```python
from build123d import *

# Parameters (mm, degrees)
SKETCH1_W           = 17.5768
SKETCH1_H           = 11.176
BOSS_EXTRUDE1_DEPTH = 24.13
CUT_EXTRUDE1_DEPTH  = 22.55
SKETCH3_W           = 2.3304
SKETCH3_H           = 3.81
SKETCH3_W_2         = 2.2288
SKETCH3_H_2         = 3.7084
CUT_EXTRUDE2_DEPTH  = 0.254


with BuildPart() as part:
    # Sketch1 → Boss-Extrude1 (new body)
    with BuildSketch(Plane.XY):
        with Locations((8.7884, 5.588)):
            Rectangle(SKETCH1_W, SKETCH1_H)
    extrude(amount=-BOSS_EXTRUDE1_DEPTH)

    # Sketch2 → Cut-Extrude1 (cut)
    with BuildSketch(Plane.XY):
        Polygon((2.8384, 1.628), (14.7384, 1.628), (14.7384, 8.228), (11.9634, 8.228), (11.9634, 9.098), (10.8184, 9.098), (10.8184, 9.548), (6.7584, 9.548), (6.7584, 9.098), (5.6134, 9.098), (5.6134, 8.228), (2.8384, 8.228), align=None)
    extrude(amount=-CUT_EXTRUDE1_DEPTH, mode=Mode.SUBTRACT)

    # Sketch3 → Cut-Extrude2 (cut)
    with BuildSketch(Plane.XY):
        with Locations((1.4192, 8.636)):
            Rectangle(SKETCH3_W, SKETCH3_H)
        with Locations((1.4192, 8.636)):
            Rectangle(SKETCH3_W_2, SKETCH3_H_2, mode=Mode.SUBTRACT)
        with Locations((16.1576, 8.636)):
            Rectangle(SKETCH3_W, SKETCH3_H)
        with Locations((16.1576, 8.636)):
            Rectangle(SKETCH3_W_2, SKETCH3_H_2, mode=Mode.SUBTRACT)
    extrude(amount=-CUT_EXTRUDE2_DEPTH, mode=Mode.SUBTRACT)


solid = part.part
```
Source: CAD feature listing. Evaluate the final solid. Frame: model axes, mm. A direction names the side the tool comes from. Coordinates: 2 decimals unless noted, no trailing zeros. Order: outer loops, then holes, each group sorted by start corner. A loop starts at its lowest first (then second) coordinate and runs counter-clockwise, first axis right, second up. Notation, with made-up numbers: (12, 0) - (52, 0) arc R15 cw to (52, 15) - close; hole circle Ø1 at (4, -12). An arc over 180 degrees is marked (long way). One line per item, written item: value.
1) Ray query, line 1 (Y direction, x = 8.75, z = -8); line 2 (Y direction, x = 12.75, z = -17.5); line 3 (X direction, y = 5.5, z = -18.5). Return the intervals inside material, ascending. Write a range as [from, to].
Computed values:
line 1: y = [0, 1.63], [9.55, 11.18]
line 2: y = [0, 1.63], [8.23, 11.18]
line 3: x = [0, 2.84], [14.74, 17.58]
2) Cut plane A-A on z = -20.25. Output: boundary loops of the cut face in (x, y).
Computed values:
outline: (0, 0) - (17.58, 0) - (17.58, 11.18) - (0, 11.18) - close; hole (2.84, 1.63) - (14.74, 1.63) - (14.74, 8.23) - (11.96, 8.23) - (11.96, 9.1) - (10.82, 9.1) - (10.82, 9.55) - (6.76, 9.55) - (6.76, 9.1) - (5.61, 9.1) - (5.61, 8.23) - (2.84, 8.23) - close
3) Cut plane B-B on y = 8.5. Output: boundary loops of the cut face in (x, z).
Computed values:
outline: (0, -24.13) - (17.58, -24.13) - (17.58, 0) - (17.32, 0) - (17.32, -0.25) - (17.27, -0.25) - (17.27, 0) - (15.04, 0) - (15.04, -0.25) - (14.99, -0.25) - (14.99, 0) - (11.96, 0) - (11.96, -22.55) - (5.61, -22.55) - (5.61, 0) - (2.58, 0) - (2.58, -0.25) - (2.53, -0.25) - (2.53, 0) - (0.3, 0) - (0.3, -0.25) - (0.25, -0.25) - (0.25, 0) - (0, 0) - close
4) Cut plane D-D on y = 2.5. Output: boundary loops of the cut face in (x, z), plus the area to 3 significant figures.
Computed values:
outline: (0, -24.13) - (17.58, -24.13) - (17.58, 0) - (14.74, 0) - (14.74, -22.55) - (2.84, -22.55) - (2.84, 0) - (0, 0) - close
area: 156 mm^2
5) Reachability of faces 4 (the face through (16, 9, 0)), 5 (the face through (2.838, 5, -11)) from +Z, -Z, +X, -X, +Y, -Y: full face, straight path, thin tool, end or side. Return the list, or none.
Computed values:
face 4: +Z, +X, -X, +Y, -Y
face 5: +Z
6) Cut plane C-C on x = 11.5. Output: boundary loops of the cut face in (y, z).
Computed values:
outline: (0, -24.13) - (11.18, -24.13) - (11.18, 0) - (9.1, 0) - (9.1, -22.55) - (1.63, -22.55) - (1.63, 0) - (0, 0) - close
7) Mould query, pull axis Y, two halves, no side actions, for faces 1 (the face through (9, 0, -12)), 2 (the face through (9, 1.628, -11)), 3 (the face through (9, 6, -24.13)). Classes: released by +Y, released by -Y, zero draft, split by the parting line, or undercut.
Computed values:
face 1: released by -Y
face 2: undercut
face 3: zero draft
